Autodesk Inventor part; units mm, degrees
ref_plane "YZ Plane" through (0, 0, 0) normal (1, 0, 0) x (0, 1, 0)
ref_plane "XZ Plane" through (0, 0, 0) normal (0, 1, 0) x (-1, 0, 0)
ref_plane "XY Plane" through (0, 0, 0) normal (0, 0, 1) x (1, 0, 0)
sketch "Sketch1" plane through (0, 0, 0) normal (0, 0, 1) x (1, 0, 0)
  line L0 (-1.283, 24.9016) -> (-1.283, -22.4465)
  line L1 (23.717, 4.5) -> (23.717, -4.5)
  line L2 (23.717, -4.5) -> (18.717, -4.5)
  line L3 (18.717, -4.5) -> (18.717, -2)
  line L4 (18.717, -2) -> (2.717, -2)
  line L5 (23.717, 4.5) -> (18.717, 4.5)
  line L6 (18.717, 4.5) -> (18.717, 2)
  line L7 (18.717, 2) -> (2.717, 2)
  line L8 (2.717, 2) -> (2.717, -2)
  line L9 (23.717, 3) -> (21.717, 1.8453)
  line L10 (21.717, 1.8453) -> (21.717, -1.8453)
  line L11 (21.717, -1.8453) -> (23.717, -3)
  point P0 (0, 0)
  point P1 (18.717, 3.25)
  point P2 (18.717, -3.25)
  point P3 (2.717, 0)
  dimension "d0" = 50
  dimension "d1" = 8
  dimension "d2" = 5
  dimension "d3" = 9
  dimension "d4" = 1.5
  dimension "d5" = 1.5
  dimension "d6" = 60
  dimension "d7" = 2
  dimension "d20" = 4
revolve "Revolution1" add sketch "Sketch1" angle 360 about axis through (-1.283, 24.9016, 0) along (0, -1, 0) contours L1 L9 L10 L11 L2 L3 L4 L8 L7 L6 L5
sketch "Sketch2" plane through (-1.283, 2, 0) normal (0, 1, 0) x (1, 0, 0)
  circle A0 centre (0, 0) radius 12 construction
  circle A1 centre (0, -12) radius 5
  circle A2 centre (11.4127, -3.7082) radius 5
  circle A3 centre (0, 0) radius 12 construction
  circle A4 centre (7.0534, 9.7082) radius 5
  circle A5 centre (0, 0) radius 12 construction
  circle A6 centre (-7.0534, 9.7082) radius 5
  circle A7 centre (0, 0) radius 12 construction
  circle A8 centre (-11.4127, -3.7082) radius 5
  circle A9 centre (0, 0) radius 12 construction
  point P0 (1.283, 0)
  dimension "d9" = 24
  dimension "d10" = 10
  dimension "d13" = 360
extrude "Extrusion1" cut sketch "Sketch2" against normal through all
sketch "Sketch3" plane through (-1.283, 2, 0) normal (0, 1, 0) x (1, 0, 0)
  circle A0 centre (0, 0) radius 5
  circle A1 centre (0, 0) radius 4
  point P0 (1.283, 0)
  dimension "d17" = 10
extrude "Extrusion2" add sketch "Sketch3" along normal blind 0.5
mirror "Mirror1" about plane through (0, 0, 0) normal (0, 1, 0) of "Extrusion2"
sketch "Sketch4" plane through (-1.283, -2.5, 0) normal (0, -1, 0) x (1, 0, 0)
  circle A0 centre (0, 0) radius 4
  circle A1 centre (-4, 0) radius 0.5
  point P0 (1.283, 0)
  point P1 (-3.9688, -0.499)
  point P2 (-3.9688, 0.499)
  dimension "d21" = 1
  dimension "d22" = 4
extrude "Extrusion3" cut sketch "Sketch4" against normal through all contours A0 A1 picked at (-4.1643, 0)
properties part number "Pulley lớn" material "Iron, Cast"
Work out the finished part from the listing and answer in its coordinate system (mm). A direction names the side the tool comes from. Give positions to 0.01 mm unless a question says otherwise; leave off trailing zeros. Write each loop counter-clockwise with the first axis right and the second up, starting at its lowest first coordinate (ties: lowest second). Pieces come first, ordered by that corner, then holes. Notation, with made-up numbers: (-10, -33) - (9, -33) arc R32 ccw to (9, 6) - close; hole circle Ø4 at (34, 86). An arc over 180 degrees is marked (long way). One line per item, written item: value. Start each with the question number.
1. Find section B-B (x = -11.5). State how many separate pieces and enclosed holes the cut face has, then the cut area to 3 significant figures.
2. Given pin 1 (11.5 mm diameter, centred on x = 10.13, z = 3.71, fed in from -Y); pin 2 (5 mm diameter, centred on y = 0.5, z = 9.5, fed in from +X); pin 3 (11.5 mm diameter, centred on x = -12.7, z = 3.71, fed in from +Y), each flat-ended and moving along its own axis, determine where each tip first touches the part or whether it passes through.
3. For a pull along X with two mould halves and no side action, classify faces 5 (the cylindrical face through (22.563, -3.761, 7.509)), 6 (the cylindrical face through (-8.987, 0.028, -14.666)), 7 (the flat face through (-13, 4.5, 17)) as +X half, -X half, draft (parallel to the pull), parting line (faces both ways), or undercut.
4. Find section A-A (y = -0.5). Write down the section's boundary in (x, z).
5. For faces 1 (the cylindrical face through (1.4, 0.03, 7.78)), 2 (the cylindrical face through (3.486, -2.246, -1.502)), 3 (the cylindrical face through (17.793, 3.232, 6.007)), 4 (the cylindrical face through (11.082, -0.026, 19.394)), determine the directions among +Z, -Z, +X, -X, +Y, -Y from which every point of the face is accessible in a straight line to the end or side of a thin tool.
6. Consider probe 1 along Z at (x, y) = (-1, 1.25); probe 2 along Z at (x, y) = (2, -0.5); probe 3 along Z at (x, y) = (-5.5, -2.25). Determine where each line is inside the solid, lowest interval first.
Geometry results:
1. separate pieces: 3
1. enclosed holes: 0
1. area: 148 mm2
2. pin 1: y = -2
2. pin 2: x = 21.95
2. pin 3: y = 2
3. face 5: parting line
3. face 6: undercut
3. face 7: draft
4. outline: circle Ø46 at (-1.28, 0); hole circle Ø10 at (-12.7, 3.71); hole circle Ø10 at (-8.34, -9.71); hole circle Ø10 at (-1.28, 12); hole (-5.25, -0.5) arc R4 ccw (long way) to (-5.25, 0.5) arc R0.5 ccw (long way) to start; hole circle Ø10 at (5.77, -9.71); hole circle Ø10 at (10.13, 3.71)
5. face 1: +Y, -Y
5. face 2: -Y
5. face 3: +Y
5. face 4: none
6. probe 1: -23 to -3.99, 3.99 to 7.01, 16.99 to 23
6. probe 2: -22.76 to -12.99, -6.42 to -2.29, 2.29 to 8.23, 15.77 to 22.76
6. probe 3: -23.32 to -19.55, -2.69 to -0.45, 0.45 to 2.69, 19.55 to 23.32
